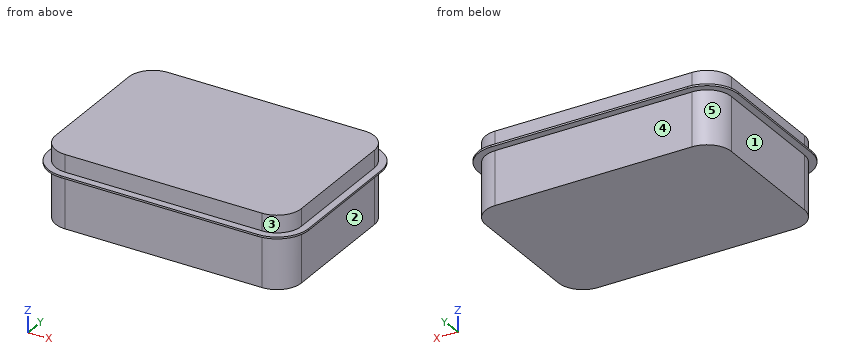
```python
from build123d import *

# Parameters (mm, degrees)
F1_DEPTH = 2.5
F2_DEPTH = 50
F3_DEPTH = 150


with BuildPart() as f1:
    # F0 (on Top) → F1 (new body, symmetric)
    with BuildSketch(Plane.XY):
        with BuildLine():
            Line((-270.5, -251), (270.5, -251))
            ThreePointArc((270.5, -251), (332.01829, -225.51829), (357.5, -164))
            Line((357.5, -164), (357.5, 164))
            ThreePointArc((357.5, 164), (332.01829, 225.51829), (270.5, 251))
            Line((270.5, 251), (-270.5, 251))
            ThreePointArc((-270.5, 251), (-332.01829, 225.51829), (-357.5, 164))
            Line((-357.5, 164), (-357.5, -164))
            ThreePointArc((-357.5, -164), (-332.01829, -225.51829), (-270.5, -251))
        make_face()
        with BuildLine():
            ThreePointArc((337.5, -164), (317.876154, -211.376154), (270.5, -231))
            Line((270.5, -231), (-270.5, -231))
            ThreePointArc((-270.5, -231), (-317.876154, -211.376154), (-337.5, -164))
            Line((-337.5, -164), (-337.5, 164))
            ThreePointArc((-337.5, 164), (-317.876154, 211.376154), (-270.5, 231))
            Line((-270.5, 231), (270.5, 231))
            ThreePointArc((270.5, 231), (317.876154, 211.376154), (337.5, 164))
            Line((337.5, 164), (337.5, -164))
        make_face(mode=Mode.SUBTRACT)
    extrude(amount=F1_DEPTH, both=True)

    # F0 (on Top) → F2 (join)
    with BuildSketch(Plane.XY):
        with BuildLine():
            Line((-270.5, -231), (270.5, -231))
            ThreePointArc((270.5, -231), (317.876154, -211.376154), (337.5, -164))
            Line((337.5, -164), (337.5, 164))
            ThreePointArc((337.5, 164), (317.876154, 211.376154), (270.5, 231))
            Line((270.5, 231), (-270.5, 231))
            ThreePointArc((-270.5, 231), (-317.876154, 211.376154), (-337.5, 164))
            Line((-337.5, 164), (-337.5, -164))
            ThreePointArc((-337.5, -164), (-317.876154, -211.376154), (-270.5, -231))
        make_face()
    extrude(amount=F2_DEPTH)

    # F0 (on Top) → F3 (join)
    with BuildSketch(Plane.XY):
        with BuildLine():
            Line((-270.5, -231), (270.5, -231))
            ThreePointArc((270.5, -231), (317.876154, -211.376154), (337.5, -164))
            Line((337.5, -164), (337.5, 164))
            ThreePointArc((337.5, 164), (317.876154, 211.376154), (270.5, 231))
            Line((270.5, 231), (-270.5, 231))
            ThreePointArc((-270.5, 231), (-317.876154, 211.376154), (-337.5, 164))
            Line((-337.5, 164), (-337.5, -164))
            ThreePointArc((-337.5, -164), (-317.876154, -211.376154), (-270.5, -231))
        make_face()
    extrude(amount=-F3_DEPTH)


solid = f1.part
```
Geometry check sheet. Reference: the model listing, model coordinates, mm. Face numbers are marked on the shaded views. A direction names the side the tool comes from. Coordinates: 2 decimals unless noted, no trailing zeros. Write each loop counter-clockwise with the first axis right and the second up, starting at its lowest first coordinate (ties: lowest second). Pieces come first, ordered by that corner, then holes. Notation, with made-up numbers: M -36,62 L -6,62 A14 cw -6,72 Z; hole C -26,-39.75 d2. An arc over 180 degrees is marked long. One line per item, written item: value. Start each with the question number.
(1) Sectioned sample at B-B, the plane x = -60. Enter the section's corners in (y, z), and give its area (3 significant figures).
(2) Scan lines: line 1 along Y through (x, z) = (-263, -103); line 2 along X through (y, z) = (-58.5, -94.5); line 3 along Y through (x, z) = (-290, -120). Record each from-to range of solid material in increasing order. Write a range as [from, to].
(3) Sectioned sample at C-C, the plane y = -137.5. Enter the section's corners in (x, z), and give its area (3 significant figures).
(4) Depth check by flat-ended pin: pin 1 (5 mm diameter, centred on y = 163, z = -82, fed in from -X); pin 2 (3 mm diameter, centred on x = -146.5, z = -74, fed in from -Y); pin 3 (4 mm diameter, centred on x = -95.5, z = -108, fed in from +Y). Enter the tip coordinate at first touch or a pass-through.
(5) Tool access check on the marked faces 1, 2, 3, 4 and 5. Record the directions out of +Z, -Z, +X, -X, +Y, -Y that give a thin tool (end or side, any length) a straight path to the whole face; none if there is none.
(6) Sectioned sample at A-A, the plane z = -75.5. Enter the section's corners in (x, y), and give its area (3 significant figures).
Filled sheet:
1. outline: M -251,-2.5 L -231,-2.5 L -231,-150 L 231,-150 L 231,-2.5 L 251,-2.5 L 251,2.5 L 231,2.5 L 231,50 L -231,50 L -231,2.5 L -251,2.5 Z
1. area: 92,600 mm²
2. line 1: [-231, 231]
2. line 2: [-337.5, 337.5]
2. line 3: [-228.1, 228.1]
3. outline: M -357.5,-2.5 L -337.5,-2.5 L -337.5,-150 L 337.5,-150 L 337.5,-2.5 L 357.5,-2.5 L 357.5,2.5 L 337.5,2.5 L 337.5,50 L -337.5,50 L -337.5,2.5 L -357.5,2.5 Z
3. area: 135,000 mm²
4. pin 1: x = -337.5
4. pin 2: y = -231
4. pin 3: y = 231
5. face 1: -Z, -X, +Y, -Y
5. face 2: -Z, +X, +Y, -Y
5. face 3: +Z, +X, -Y
5. face 4: -Z, +X, -X, +Y
5. face 5: -Z, -X, +Y
6. outline: M -337.5,-164 A67 ccw -270.5,-231 L 270.5,-231 A67 ccw 337.5,-164 L 337.5,164 A67 ccw 270.5,231 L -270.5,231 A67 ccw -337.5,164 Z
6. area: 308,000 mm²
